Design review of the part shown in the three views and the two pictorial views. Dimensions are in mm from the part's minimum x, y and z. A direction names the side the tool comes from. Give positions to 0.01 mm unless a question says otherwise; leave off trailing zeros. Loops run counter-clockwise (first coordinate to the right, second up) from the corner with the lowest first, then second, coordinate; pieces in that order, holes last. Notation, with made-up numbers: (-19, 20.25) - (37, 20.25) arc R33 ccw to (37, 57.25) - close; hole circle Ø8 at (-35, 8). An arc over 180 degrees is marked (long way). Use CSV: the item, a comma, the result in double quotes. Start each with the question number.
1. Take a section at C-C on z = 26.5. Give the boundary of the cut face in (x, y).
2. For the marked faces 5 and 6, list the 3-axis set-ups (+Z, -Z, +X, -X, +Y, -Y) from which the entire face can be reached by the end or side of a thin tool; tool diameter is ignored.
3. Take a section at A-A on y = 10. Give the boundary of the cut face in (x, z).
4. For pin 1 (3 mm diameter, centred on x = 16.8, z = 12, fed in from +Y); pin 2 (0.6 mm diameter, centred on x = 19.5, z = 1, fed in from +Y); pin 3 (8 mm diameter, centred on x = 26.5, y = 16, fed in from -Z), all flat-tipped, find the tip position at first contact; note any pin that passes through.
5. Wall thickness on line 1 (X direction, y = 1, z = 22); line 2 (Z direction, x = 16.8, y = 1.45); line 3 (Z direction, x = 37, y = 13.5): over which ranges is each line inside the solid? List them lowest first.
6. Take a section at B-B on x = 32.5. Give the boundary of the cut face in (y, z).
7. Mouldability with a two-part tool opening along Z and no side actions: class the marked faces 1, 2, 3 and 4 as pulls with the +Z half, pulls with the -Z half, needs draft (parallel to the pull), parting line crosses it, or undercut.
8. Take a section at D-D on x = 9. Give the boundary of the cut face in (y, z).
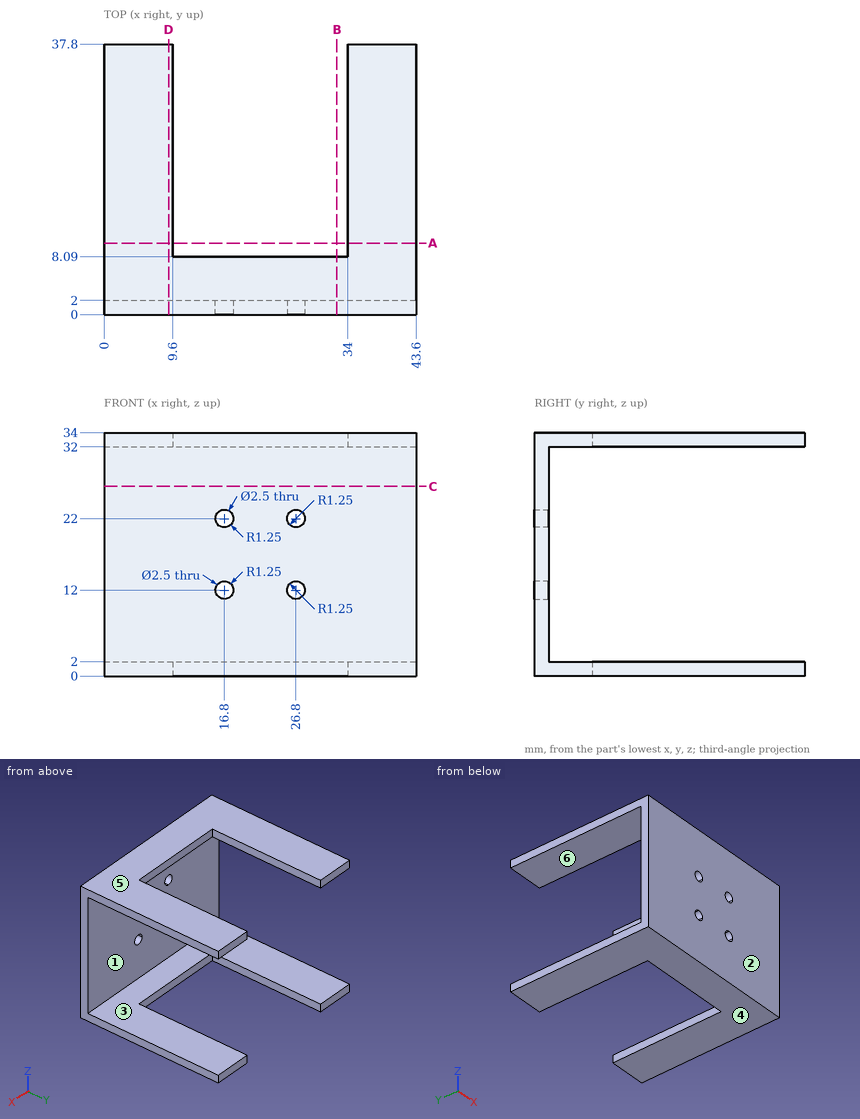
Check result:
1,outline,"(0, 0) - (43.6, 0) - (43.6, 2) - (0, 2) - close"
2,face 5,"+Z, +X, -X, +Y, -Y"
2,face 6,"+X, -X, +Y"
3,outline,"(0, 0) - (9.6, 0) - (9.6, 2) - (0, 2) - close; (0, 32) - (9.6, 32) - (9.6, 34) - (0, 34) - close; (34, 0) - (43.6, 0) - (43.6, 2) - (34, 2) - close; (34, 32) - (43.6, 32) - (43.6, 34) - (34, 34) - close"
4,pin 1,"stops at y = 2"
4,pin 2,"stops at y = 8.09"
4,pin 3,"passes through"
5,line 1,"x = 0 to 15.55, 18.05 to 25.55, 28.05 to 43.6"
5,line 2,"z = 0 to 10.75, 13.25 to 20.75, 23.25 to 34"
5,line 3,"z = 0 to 2, 32 to 34"
6,outline,"(0, 0) - (8.09, 0) - (8.09, 2) - (2, 2) - (2, 32) - (8.09, 32) - (8.09, 34) - (0, 34) - close"
7,face 1,"undercut"
7,face 2,"needs draft"
7,face 3,"undercut"
7,face 4,"pulls with the -Z half"
8,outline,"(0, 0) - (37.8, 0) - (37.8, 2) - (2, 2) - (2, 32) - (37.8, 32) - (37.8, 34) - (0, 34) - close"
